from build123d import *

# Parameters (mm, degrees)
SKETCH1_R           = 1.572651685
SKETCH1_W           = 11.644038646
SKETCH1_H           = 5.765279756
SKETCH1_R_2         = 1.5875
SKETCH1_R_3         = 1.573453894
SKETCH1_R_4         = 1.559986851
SKETCH1_R_5         = 6.598413588
SKETCH1_R_6         = 1.572849618
SKETCH1_R_7         = 1.499975878
SKETCH1_R_8         = 1.537647246
SKETCH1_W_2         = 4.506321673
SKETCH1_H_2         = 21.672357955
SKETCH1_R_9         = 1.455342512
BOSS_EXTRUDE1_DEPTH = 4


with BuildPart() as part:
    # Sketch1 → Boss-Extrude1 (new body)
    with BuildSketch(Plane(origin=(0, 0, 0), x_dir=(1, 0, 0), z_dir=(0, 1, 0))):
        with BuildLine():
            Line((80, 43.971671866), (80, 53))
            Line((80, 53), (-80, 53))
            Line((-80, 53), (-80, 43.971671866))
            add(Edge.make_bspline(
                [(-80, 43.971671866), (-65.385653613, 39.40479143), (-89.077453909, 33.627557401), (-66.52691334, 21.603012731), (-80, 18.948157225)],
                knots=[0, 0, 0, 0, 0.464080818, 1, 1, 1, 1], degree=3))
            Line((-80, 18.948157225), (-80, 11.773195968))
            ThreePointArc((-80, 11.773195968), (-71.103660502, -0.526648314), (-80, -12.826492596))
            Line((-80, -12.826492596), (-80, -16.469279615))
            Line((-80, -16.469279615), (-80, -18.948157225))
            add(Edge.make_bspline(
                [(-80, -43.971671866), (-65.385653613, -39.40479143), (-89.077453909, -33.627557401), (-66.52691334, -21.603012731), (-80, -18.948157225)],
                knots=[0, 0, 0, 0, 0.464080818, 1, 1, 1, 1], degree=3))
            Line((-80, -43.971671866), (-80, -48.36784463))
            Line((-80, -48.36784463), (-80, -53))
            Line((-80, -53), (80, -53))
            Line((80, -53), (80, -43.971671866))
            add(Edge.make_bspline(
                [(80, -43.971671866), (65.385653613, -39.40479143), (89.077453909, -33.627557401), (66.52691334, -21.603012731), (80, -18.948157225)],
                knots=[0, 0, 0, 0, 0.464080818, 1, 1, 1, 1], degree=3))
            Line((80, -18.948157225), (80, -12.826492596))
            ThreePointArc((80, -12.826492596), (71.103660502, -0.526648314), (80, 11.773195968))
            Line((80, 11.773195968), (80, 18.948157225))
            add(Edge.make_bspline(
                [(80, 43.971671866), (65.385653613, 39.40479143), (89.077453909, 33.627557401), (66.52691334, 21.603012731), (80, 18.948157225)],
                knots=[0, 0, 0, 0, 0.464080818, 1, 1, 1, 1], degree=3))
        make_face()
        with Locations(Location((-62.250436779, -43.20843745, 0), (0, 0, 270))):
            Circle(SKETCH1_R, mode=Mode.SUBTRACT)
        with Locations(Location((-25.714592034, -43.20843745, 0), (0, 0, 270))):
            Circle(SKETCH1_R, mode=Mode.SUBTRACT)
        with Locations((-12.847001436, -26.953726478)):
            Rectangle(SKETCH1_W, SKETCH1_H, mode=Mode.SUBTRACT)
        with Locations(Location((-62.250436779, -6.647294825, 0), (0, 0, 270))):
            Circle(SKETCH1_R, mode=Mode.SUBTRACT)
        with Locations(Location((-25.714592034, -6.647294825, 0), (0, 0, 270))):
            Circle(SKETCH1_R, mode=Mode.SUBTRACT)
        with Locations(Location((9.080460795, -32.68, 0), (0, 0, 270))):
            Circle(SKETCH1_R_2, mode=Mode.SUBTRACT)
        with BuildLine():
            ThreePointArc((4.499768913, -37.552295579), (0, -42.052064492), (-4.499768913, -37.552295579))
            Line((-4.499768913, -37.552295579), (-4.499768913, -16.469279615))
            ThreePointArc((-4.499768913, -16.469279615), (0, -11.969510703), (4.499768913, -16.469279615))
            Line((4.499768913, -16.469279615), (4.499768913, -37.552295579))
        make_face(mode=Mode.SUBTRACT)
        with Locations(Location((57.340460795, -31.41, 0), (0, 0, 270))):
            Circle(SKETCH1_R_2, mode=Mode.SUBTRACT)
        with Locations(Location((-62.250436779, 2.210073291, 0), (0, 0, 270))):
            Circle(SKETCH1_R_3, mode=Mode.SUBTRACT)
        with Locations(Location((-25.714592034, 2.210073291, 0), (0, 0, 270))):
            Circle(SKETCH1_R_4, mode=Mode.SUBTRACT)
        with Locations(Location((-4.725453474, 0, 0), (0, 0, 270))):
            Circle(SKETCH1_R_5, mode=Mode.SUBTRACT)
        with BuildLine():
            ThreePointArc((4.499768913, 14.833404805), (6.242806414, 13.090367304), (4.499768913, 11.347329803))
            Line((4.499768913, 11.347329803), (-13.950675862, 11.347329803))
            ThreePointArc((-13.950675862, 11.347329803), (-15.693713363, 13.090367304), (-13.950675862, 14.833404805))
            Line((-13.950675862, 14.833404805), (4.499768913, 14.833404805))
        make_face(mode=Mode.SUBTRACT)
        with Locations(Location((-62.250436779, 38.687345787, 0), (0, 0, 270))):
            Circle(SKETCH1_R_6, mode=Mode.SUBTRACT)
        with BuildLine():
            add(Edge.make_bspline(
                [(-39.652356334, 45.238000012), (-39.652356334, 48.238000012), (-42.652356334, 48.238000012), (-42.652356334, 45.238000012), (-42.652356334, 42.238000012), (-39.652356334, 42.238000012), (-39.652356334, 45.238000012)],
                knots=[0, 0, 0, 0, 0.5, 0.5, 0.5, 1, 1, 1, 1], degree=3, weights=[1, 0.333333333, 0.333333333, 1, 0.333333333, 0.333333333, 1]))
        make_face(mode=Mode.SUBTRACT)
        with Locations(Location((-25.714592034, 38.687345787, 0), (0, 0, 270))):
            Circle(SKETCH1_R_7, mode=Mode.SUBTRACT)
        Polygon((0.058166934, 21.830550018), (-8.655922933, 21.598581172), (-13.21385878, 29.029219944), (-9.05770476, 36.691827563), (-0.343614893, 36.923796409), (4.214320954, 29.493157636), align=None, mode=Mode.SUBTRACT)
        with Locations(Location((14.160460795, 19.39, 0), (0, 0, 270))):
            Circle(SKETCH1_R_2, mode=Mode.SUBTRACT)
        with Locations(Location((14.894900679, 24.261040082, 0), (0, 0, 270))):
            Circle(SKETCH1_R_8, mode=Mode.SUBTRACT)
        with Locations(Location((42.100460795, 19.39, 0), (0, 0, 270))):
            Circle(SKETCH1_R_2, mode=Mode.SUBTRACT)
        with Locations((54.219607529, 37.531665653)):
            Rectangle(SKETCH1_W_2, SKETCH1_H_2, mode=Mode.SUBTRACT)
        with Locations(Location((45.983391129, 40.924373364, 0), (0, 0, 270))):
            Circle(SKETCH1_R_9, mode=Mode.SUBTRACT)
        with BuildLine():
            add(Edge.make_bspline(
                [(47.342643666, 45.238000012), (47.342643666, 48.238000012), (44.342643666, 48.238000012), (44.342643666, 45.238000012), (44.342643666, 42.238000012), (47.342643666, 42.238000012), (47.342643666, 45.238000012)],
                knots=[0, 0, 0, 0, 0.5, 0.5, 0.5, 1, 1, 1, 1], degree=3, weights=[1, 0.333333333, 0.333333333, 1, 0.333333333, 0.333333333, 1]))
        make_face(mode=Mode.SUBTRACT)
    extrude(amount=BOSS_EXTRUDE1_DEPTH)


solid = part.part
The model under review builds one solid part; all positions refer to its coordinate system, in mm. A direction names the side the tool comes from. Coordinates: 2 decimals unless noted, no trailing zeros.
(1) Wall thickness on L1, parallel to Z at x = -15, y = 0.6; L2, parallel to X at y = 2.85, z = 0; L3, parallel to Z at x = -8.5, y = 2.35: over which ranges is each line inside the solid? List them lowest first.
Determined:
L1: z = -53 to -14.48, -11.7 to 24.07, 29.84 to 53
L2: x = -71.11 to -11.32, 1.87 to 71.11
L3: z = -53 to -36.71, -21.6 to -14.83, -11.35 to -5.41, 5.41 to 24.07, 29.84 to 53
(2) Consider section A-A, the plane y = 1.25. Give the number of separate pieces and of enclosed holes in the cut face, plus the area to 3 significant figures.
Determined:
separate pieces: 1
enclosed holes: 22
area: 15,200 mm2
(3) Tool access review of faces 4 (the flat face through (-13, 2, 29.836)), 5 (the flat face through (80, 2, -15)): name each direction out of +Z, -Z, +X, -X, +Y, -Y from which nothing blocks a thin tool from reaching the whole face with its end or side.
Determined:
face 4: +Y, -Y
face 5: +Z, -Z, +X, +Y, -Y
(4) Insertion check: P1, Ø1, axis at y = 2.5, z = -32.5, coming from the -X side; P2, Ø1.2, axis at y = 1, z = 29.5, coming from the -X side. Each pin has a flat end and moves straight along its axis. Give the tip position at first contact, or say it passes through.
Determined:
P1: stops at x = -77.5
P2: stops at x = -77.02
(5) Draft analysis for pull direction X (two halves, no side actions). For faces 1 (the cylindrical face through (13.53, 1.97, -23.55)), 2 (the flat face through (-1, 0, 11)), 3 (the cylindrical face through (71.106, 1.972, 0.754)), state which applies: +X half, -X half, draft (parallel to the pull), parting line (faces both ways), or undercut.
Determined:
face 1: undercut
face 2: draft
face 3: +X half
